Geometry check sheet. Reference: the model listing, model coordinates, mm. Coordinates: 2 decimals unless noted, no trailing zeros. Order: outer loops, then holes, each group sorted by start corner. A loop starts at its lowest first (then second) coordinate and runs counter-clockwise, first axis right, second up. Notation, with made-up numbers: (-36.75, 24.5) - (-4.75, 24.5) arc R11 cw to (-4.75, 36.5) - close; hole circle Ø3 at (-8, 87). An arc over 180 degrees is marked (long way). Put each result on its own line as item: value.
from build123d import *

# Parameters (mm, degrees)
SKETCH_1_W          = 10
SKETCH_1_H          = 160
EXTRUDE_1_DEPTH     = 10
SKETCH_3_W          = 10
SKETCH_3_H          = 10
CUT_EXTRUDE_1_DEPTH = 5
HOLE_WIZARD_M4_1_D  = 3.3
SKETCH_7_R          = 3.25
CUT_EXTRUDE_2_DEPTH = 1


with BuildPart() as part:
    # 草图1 → 凸台-拉伸1 (new body)
    with BuildSketch(Plane.XY):
        with Locations((5, -80)):
            Rectangle(SKETCH_1_W, SKETCH_1_H)
    extrude(amount=EXTRUDE_1_DEPTH)

    # 草图3 → 切除-拉伸1 (cut)
    with BuildSketch(Plane(origin=(0, 0, 0), x_dir=(-1, 0, 0), z_dir=(0, 0, -1))):
        with Locations((-5, -5)):
            Rectangle(SKETCH_3_W, SKETCH_3_H)
        with Locations((-5, -155)):
            Rectangle(SKETCH_3_W, SKETCH_3_H)
    extrude(amount=-CUT_EXTRUDE_1_DEPTH, mode=Mode.SUBTRACT)

    # M4 螺纹孔的螺纹孔钻头1 (through all)
    with Locations(Plane.XY.offset(10)):
        with Locations((5, -5), (5, -155)):
            Hole(HOLE_WIZARD_M4_1_D / 2)

    # 草图7 → 切除-拉伸2 (cut)
    with BuildSketch(Plane.XY.offset(10)):
        with Locations((5, -5)):
            Circle(SKETCH_7_R)
        with Locations((5, -155)):
            Circle(SKETCH_7_R)
    extrude(amount=-CUT_EXTRUDE_2_DEPTH, mode=Mode.SUBTRACT)


solid = part.part
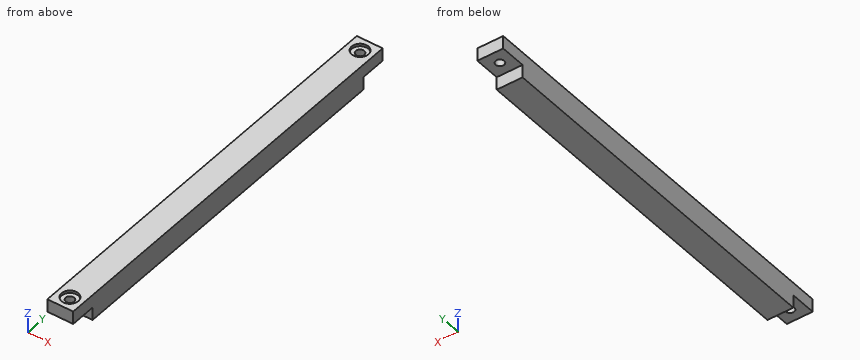
Q1. Thickness scan on L1, parallel to Y at x = 5, z = 8.2; L2, parallel to Y at x = 5, z = 9.7; L3, parallel to X at y = -155, z = 9.65. Record the ranges inside material, lowest first. Write a range as [from, to].
Answer block:
L1: y = [-160, -156.65], [-153.35, -6.65], [-3.35, 0]
L2: y = [-160, -158.25], [-151.75, -8.25], [-1.75, 0]
L3: x = [0, 1.75], [8.25, 10]
Q2. Section check B-B on y = -155. Record the boundary of the cut face in (x, z), then the cut area to 3 significant figures.
Answer block:
outline: (0, 5) - (3.35, 5) - (3.35, 9) - (1.75, 9) - (1.75, 10) - (0, 10) - close; (6.65, 5) - (10, 5) - (10, 10) - (8.25, 10) - (8.25, 9) - (6.65, 9) - close
area: 30.3 mm^2
Q3. Depth check by flat-ended pin: pin 1 Ø3 at (x, y) = (5, -155) entering from -Z; pin 2 Ø3 at (x, y) = (6.5, -3) entering from -Z; pin 3 Ø4.5 at (x, y) = (5, -5) entering from +Z; pin 4 Ø1.5 at (x, z) = (6.5, 3) entering from -Y. Enter the tip coordinate at first touch or a pass-through.
Answer block:
pin 1: passes through
pin 2: stops at z = 5
pin 3: stops at z = 9
pin 4: stops at y = -150
Q4. Section check C-C on z = 3. Record the boundary of the cut face in (x, y).
Answer block:
outline: (0, -150) - (10, -150) - (10, -10) - (0, -10) - close
Q5. Section check A-A on x = 5. Record the boundary of the cut face in (y, z), then the cut area to 3 significant figures.
Answer block:
outline: (-160, 5) - (-156.65, 5) - (-156.65, 9) - (-158.25, 9) - (-158.25, 10) - (-160, 10) - close; (-153.35, 5) - (-150, 5) - (-150, 0) - (-10, 0) - (-10, 5) - (-6.65, 5) - (-6.65, 9) - (-8.25, 9) - (-8.25, 10) - (-151.75, 10) - (-151.75, 9) - (-153.35, 9) - close; (-3.35, 5) - (0, 5) - (0, 10) - (-1.75, 10) - (-1.75, 9) - (-3.35, 9) - close
area: 1,460 mm^2
